Build history of the part. All positions in model axes, mm. A direction names the side the tool comes from. Coordinates: 2 decimals unless noted, no trailing zeros. Write each loop counter-clockwise with the first axis right and the second up, starting at its lowest first coordinate (ties: lowest second). Pieces come first, ordered by that corner, then holes.
```python
from build123d import *

# Parameters (mm, degrees)
EXTRUDE_583_DEPTH   = 30
EXTRUDE_631_DEPTH   = 10
FILLET_1_R          = 5
HOLE_WIZARD_M5_1_D  = 5.3
CUT_EXTRUDE_1_DEPTH = 5


with BuildPart() as part:
    # 草图1 → Extrude 583 (new body)
    with BuildSketch(Plane(origin=(0, 0, 0), x_dir=(1, 0, 0), z_dir=(0, 1, 0))):
        with BuildLine():
            Line((5.761926966, -165), (-5.761926966, -165))
            Line((-5.761926966, -165), (-6.805401857, -194.881211269))
            ThreePointArc((-6.805401857, -194.881211269), (0, -195), (6.805401857, -194.881211269))
            Line((6.805401857, -194.881211269), (5.761926966, -165))
        make_face()
    extrude(amount=EXTRUDE_583_DEPTH)

    # 草图1<3> → Extrude 631 (add)
    with BuildSketch(Plane(origin=(0, 0, 0), x_dir=(1, 0, 0), z_dir=(0, 1, 0))):
        with BuildLine():
            ThreePointArc((6.805401857, -194.881211269), (0, -195), (-6.805401857, -194.881211269))
            Line((-6.805401857, -194.881211269), (-6.979899341, -199.878165404))
            ThreePointArc((-6.979899341, -199.878165404), (0, -200), (6.979899341, -199.878165404))
            Line((6.979899341, -199.878165404), (6.805401857, -194.881211269))
        make_face()
    extrude(amount=EXTRUDE_631_DEPTH)

    # 圆角1
    fillet_1_edges = [part.edges().sort_by_distance(p)[0] for p in [
        (0, 0, 165),
        (-5.761926966, 15, 165),
        (5.761926966, 15, 165),
    ]]
    fillet(fillet_1_edges, radius=FILLET_1_R)

    # M5 间隙孔1 (through all)
    with Locations(Plane(origin=(0, 30, 0), x_dir=(1, 0, 0), z_dir=(0, 1, 0))):
        with Locations((0, -187), (0, -175)):
            Hole(HOLE_WIZARD_M5_1_D / 2)

    # 草图6 → 切除-拉伸1 (cut)
    with BuildSketch(Plane.XZ):
        Polygon((-4.67653718, 175), (-2.33826859, 170.95), (2.33826859, 170.95), (4.67653718, 175), (2.33826859, 179.05), (-2.33826859, 179.05), align=None)
        Polygon((-4.67653718, 187), (-2.33826859, 182.95), (2.33826859, 182.95), (4.67653718, 187), (2.33826859, 191.05), (-2.33826859, 191.05), align=None)
    extrude(amount=-CUT_EXTRUDE_1_DEPTH, mode=Mode.SUBTRACT)


solid = part.part
```
1. Saw through at A-A on x = 0. List the corners of the cut face in (y, z).
Computed values:
outline: (0, 170) arc R5 ccw to (5, 165) - (30, 165) - (30, 172.35) - (5, 172.35) - (5, 170.95) - (0, 170.95) - close; (0, 179.05) - (5, 179.05) - (5, 177.65) - (30, 177.65) - (30, 184.35) - (5, 184.35) - (5, 182.95) - (0, 182.95) - close; (0, 191.05) - (5, 191.05) - (5, 189.65) - (30, 189.65) - (30, 195) - (10, 195) - (10, 200) - (0, 200) - close
2. Saw through at C-C on x = -4. List the corners of the cut face in (y, z), plus the area to 3 significant figures.
Computed values:
outline: (0, 170) arc R5 ccw to (1.93, 166.05) - (30, 166.05) - (30, 194.96) - (10, 194.96) - (10, 199.96) - (0, 199.96) - (0, 188.17) - (5, 188.17) - (5, 185.83) - (0, 185.83) - (0, 176.17) - (5, 176.17) - (5, 173.83) - (0, 173.83) - close
area: 892 mm2
3. Saw through at D-D on z = 193. List the corners of the cut face in (x, y), plus the area to 3 significant figures.
Computed values:
outline: (-6.74, 0) - (6.74, 0) - (6.74, 30) - (-6.74, 30) - close
area: 404 mm2
4. Flat gauge pins, fed straight in: pin 1 (2 mm diameter, centred on y = 21, z = 176, fed in from -X); pin 2 (12 mm diameter, centred on y = 23, z = 184, fed in from +X); pin 3 (6 mm diameter, centred on y = 19, z = 185, fed in from -X); pin 4 (5 mm diameter, centred on x = 0, z = 175, fed in from +Y). Where does each tip first touch, or does it go through?
Computed values:
pin 1: stops at x = -6.18
pin 2: stops at x = 6.63
pin 3: stops at x = -6.57
pin 4: passes through
5. Probe line 1 along Z through (x, y) = (0, 13.5); line 2 along Z through (x, y) = (2, 5.5); line 3 along Y through (x, z) = (4.5, 198). List the from-to ranges inside material, lowest first.
Computed values:
line 1: z = 165 to 172.35, 177.65 to 184.35, 189.65 to 195
line 2: z = 165.12 to 173.26, 176.74 to 185.26, 188.74 to 199.99
line 3: y = 0 to 10
6. 3-axis set-ups, long thin cutter, end or side, ignore diameter. For faces 5 (the face through (3.491, 2.465, 184.947)), 6 (the face through (0, 20, 195)), 7 (the face through (0, 17, 165)): which of +Z, -Z, +X, -X, +Y, -Y reach the whole face in a straight line?
Computed values:
face 5: -Y
face 6: +Z, +Y
face 7: -Z, +X, -X, +Y, -Y
7. Mould opens along Z. For faces 1 (the face through (-3.491, 2.465, 189.053)), 2 (the face through (0, 5, 200)), 3 (the face through (0, 1, 167)), 4 (the face through (2, 5, 177)) say: +Z half, -Z half, draft (parallel to the pull), parting line (faces both ways), or undercut.
Computed values:
face 1: undercut
face 2: +Z half
face 3: -Z half
face 4: undercut
8. Saw through at B-B on y = 26.5. List the corners of the cut face in (x, z), plus the area to 3 significant figures.
Computed values:
outline: (-6.81, 194.88) - (-5.93, 169.83) arc R5 ccw to (-0.93, 165) - (0.93, 165) arc R5 ccw to (5.93, 169.83) - (6.81, 194.88) arc R195 ccw to start; hole circle Ø5.3 at (0, 175); hole circle Ø5.3 at (0, 187)
area: 323 mm2
